from build123d import *


with BuildPart() as f1:
    # F0 (on Front) → F1 (revolve)
    with BuildSketch(Plane.XZ):
        with BuildLine():
            Line((0, 28.4764673561), (-0.870731233, -48.2042273823))
            ThreePointArc((-0.870731233, -48.2042273823), (3.2356058271, -46.6364067901), (4.6311216429, -42.4683615565))
            Line((4.6311216429, -42.4683615565), (4.6311216429, 0))
            Line((4.6311216429, 0), (25.5204327404, 0))
            Line((25.5204327404, 0), (25.5204327404, 5.0252587534))
            Line((25.5204327404, 5.0252587534), (4.6311216429, 5.0252587534))
            Line((4.6311216429, 5.0252587534), (4.6311216429, 28.4764673561))
            Line((4.6311216429, 28.4764673561), (0, 28.4764673561))
        make_face()
    revolve(axis=Axis((-0.4353656165, 0, -9.8638800131), (0.0113545542, 0, 0.999935535)))


solid = f1.part
Check sheet for the modelled part. Datum: model origin and axes. Units: mm. Give positions to 0.01 mm unless a question says otherwise; leave off trailing zeros. Answer as CSV lines item,"result".
1. Scan lines: probe 1 along Z at (x, y) = (20, 6); probe 2 along Z at (x, y) = (2, -18.5); probe 3 along X at (y, z) = (7.5, 3). Record each from-to range of solid material in increasing order. Write a range as from..to.
Result sheet:
probe 1,"0.01..5.04"
probe 2,"0.19..5.21"
probe 3,"-24.99..24.41"
2. Go/stop test with flat-tipped pins: P1, Ø5, axis at x = -16, y = 10.5, coming from the +Z side; P2, Ø6, axis at x = 0, y = 15.5, coming from the +Z side; P3, Ø1.5, axis at x = 3, y = -13.5, coming from the -Z side; P4, Ø5, axis at y = -8, z = -14, coming from the -X side. Record where each tip stops, or that it passes through.
Result sheet:
P1,"z = 5.47"
P2,"z = 5.25"
P3,"z = 0.11"
P4,"through"
3. Mould release check, pull along Y, two halves, no side actions. Record for faces 1 (the face through (-1.547, -5.771, 5.107)), 2 (the face through (-1.686, -5.068, -20.865)): released by +Y, released by -Y, zero draft, split by the parting line, or undercut.
Result sheet:
face 1,"undercut"
face 2,"split by the parting line"
